Study the drawing (mm; zero at the part's minimum x, y, z) and answer. A direction names the side the tool comes from. Round coordinates to 2 decimals unless told otherwise and drop trailing zeros. Write each loop counter-clockwise with the first axis right and the second up, starting at its lowest first coordinate (ties: lowest second). Pieces come first, ordered by that corner, then holes. Notation, with made-up numbers: M 53,27.5 L 66,27.5 A33 ccw 66,65.5 Z; hole C 71.25,37.25 d9. An arc over 180 degrees is marked long. Write each question's results on one line, items separated by ' | '.
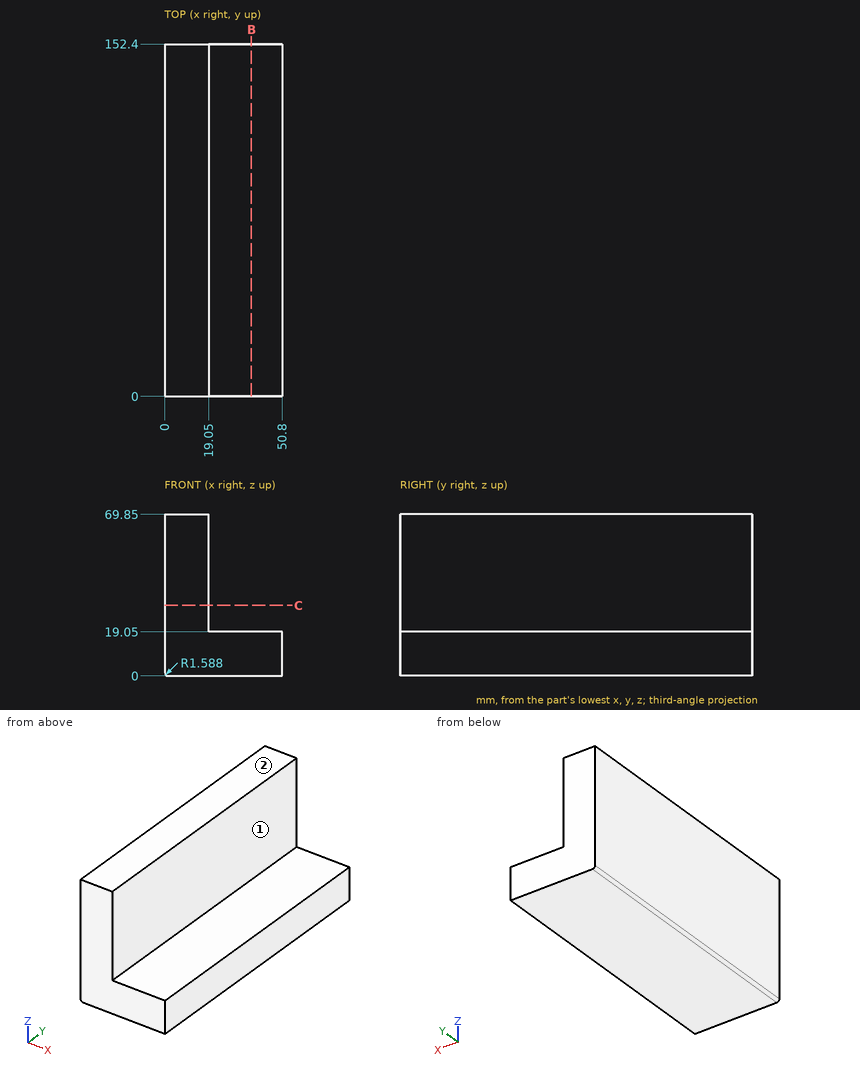
1) Find the intervals of material crossed by line 1 (X direction, y = 58, z = 56.5), in increasing order.
Return value:
line 1: 0 to 19.05
2) Each of these flat-tipped pins is pushed along its axis until it touches: pin 1 (8 mm diameter, centred on y = 36, z = 27, fed in from +X); pin 2 (10 mm diameter, centred on x = 34, y = 119.5, fed in from +Z). Where does it stop, or does it pass through?
Return value:
pin 1: x = 19.05 | pin 2: z = 19.05
3) A tool of negligible diameter and unlimited length cuts with its end or side. For the marked faces 1 and 2, from which of +Z, -Z, +X, -X, +Y, -Y can it reach the whole face along a straight path? Write none if from no direction.
Return value:
face 1: +Z, +X, +Y, -Y | face 2: +Z, +X, -X, +Y, -Y
4) Section B-B (x = 37.5) is taken. Determine the outline of the cut face in (y, z).
Return value:
outline: M 0,0 L 152.4,0 L 152.4,19.05 L 0,19.05 Z
5) Section C-C (z = 30.5) is taken. Determine the outline of the cut face in (x, y).
Return value:
outline: M 0,0 L 19.05,0 L 19.05,152.4 L 0,152.4 Z
